from build123d import *

# Parameters (mm, degrees)
SKETCH1_R           = 1.905
BOSS_EXTRUDE1_DEPTH = 9.525
SKETCH2_R           = 45.72
CUT_EXTRUDE1_DEPTH  = 12.7
SKETCH4_R           = 1.905
CUT_EXTRUDE3_DEPTH  = 12.7
CIRPATTERN2_COUNT   = 4
SKETCH10_R          = 0.6985
CUT_EXTRUDE5_DEPTH  = 3.175
CIRPATTERN5_COUNT   = 4
CHAMFER1_SIZE       = 12.7
CHAMFER1_SIZE2      = 7.332348419


with BuildPart() as part:
    # Sketch1 → Boss-Extrude1 (new body)
    with BuildSketch(Plane(origin=(0, 0, 0), x_dir=(1, 0, 0), z_dir=(0, 1, 0))):
        with BuildLine():
            ThreePointArc((-66.860826677, 58.590441679), (-88.9, 0), (-66.860826677, -58.590441679))
            ThreePointArc((-66.860826677, -58.590441679), (-65.466067123, -65.466067123), (-58.590441679, -66.860826677))
            ThreePointArc((-58.590441679, -66.860826677), (0, -88.9), (58.590441679, -66.860826677))
            ThreePointArc((58.590441679, -66.860826677), (65.466067123, -65.466067123), (66.860826677, -58.590441679))
            ThreePointArc((66.860826677, -58.590441679), (88.9, 0), (66.860826677, 58.590441679))
            ThreePointArc((66.860826677, 58.590441679), (65.466067123, 65.466067123), (58.590441679, 66.860826677))
            ThreePointArc((58.590441679, 66.860826677), (0, 88.9), (-58.590441679, 66.860826677))
            ThreePointArc((-58.590441679, 66.860826677), (-65.466067123, 65.466067123), (-66.860826677, 58.590441679))
        make_face()
        with Locations(Location((-60.975939062, 60.975939062, 0), (0, 0, 90))):
            Circle(SKETCH1_R, mode=Mode.SUBTRACT)
        with Locations(Location((60.975939062, 60.975939062, 0), (0, 0, 90))):
            Circle(SKETCH1_R, mode=Mode.SUBTRACT)
        with Locations(Location((60.975939062, -60.975939062, 0), (0, 0, 90))):
            Circle(SKETCH1_R, mode=Mode.SUBTRACT)
        with Locations(Location((-60.975939062, -60.975939062, 0), (0, 0, 90))):
            Circle(SKETCH1_R, mode=Mode.SUBTRACT)
    extrude(amount=BOSS_EXTRUDE1_DEPTH)

    # Sketch2 → Cut-Extrude1 (cut)
    with BuildSketch(Plane(origin=(0, 9.525, 0), x_dir=(1, 0, 0), z_dir=(0, 1, 0))):
        with Locations(Location((0, 0, 0), (0, 0, 270))):
            Circle(SKETCH2_R)
    extrude(amount=-CUT_EXTRUDE1_DEPTH, mode=Mode.SUBTRACT)

    # Sketch4 → Cut-Extrude3 (cut)
    with BuildSketch(Plane(origin=(0, 9.525, 0), x_dir=(1, 0, 0), z_dir=(0, 1, 0))):
        with Locations(Location((0, 82.55, 0), (0, 0, 270))):
            Circle(SKETCH4_R)
    cut_extrude3 = extrude(amount=-CUT_EXTRUDE3_DEPTH, mode=Mode.SUBTRACT)

    # CirPattern2: Cut-Extrude3 ×4 about axis
    cirpattern2_axis = Axis((0, 0, 0), (0, 1, 0))
    for i in range(1, CIRPATTERN2_COUNT):
        add(cut_extrude3.rotate(cirpattern2_axis, i * 360 / CIRPATTERN2_COUNT), mode=Mode.SUBTRACT)

    # Sketch10 → Cut-Extrude5 (cut)
    with BuildSketch(Plane(origin=(-62.861792847, 0, -62.861792847), x_dir=(0, -1, 0), z_dir=(-0.7071067811865464, 0, -0.7071067811865488))):
        with Locations(Location((-4.826, 0, 0), (0, 0, 90))):
            Circle(SKETCH10_R)
    cut_extrude5 = extrude(amount=-CUT_EXTRUDE5_DEPTH, mode=Mode.SUBTRACT)

    # CirPattern5: Cut-Extrude5 ×4 about axis
    cirpattern5_axis = Axis((0, 0, 0), (0, 1, 0))
    for i in range(1, CIRPATTERN5_COUNT):
        add(cut_extrude5.rotate(cirpattern5_axis, i * 360 / CIRPATTERN5_COUNT), mode=Mode.SUBTRACT)

    # Chamfer1
    chamfer1_edges = [part.edges().sort_by_distance(p)[0] for p in [
        (0, 9.525, -45.72),
    ]]
    chamfer1_side = [part.faces().sort_by_distance(p)[0] for p in [
        (0, 9.525, -86.385528286),
    ]]
    chamfer(chamfer1_edges, length=CHAMFER1_SIZE, length2=CHAMFER1_SIZE2, reference=chamfer1_side[0])


solid = part.part
Read the model definition and answer for the solid it produces. Units are mm, in the model's axes. Coordinates: 2 decimals unless noted, no trailing zeros. Use a Markdown table: item, result.
Q1. Straight lines are drawn through the part: L1, parallel to X at y = 6, z = 61.5; L2, parallel to Z at x = -17.5, y = 4.25; L3, parallel to Z at x = 34.5, y = 1.25. For each, find the intervals that lie inside material, in ascending order. Write a range as [from, to].
Answer block:
| item | result |
|---|---|
| L1 | x = [-67.3, -62.81], [-59.14, 59.14], [62.81, 67.3] |
| L2 | z = [-87.16, -46.07], [46.07, 87.16] |
| L3 | z = [-81.93, -30], [30, 81.93] |
Q2. Determine the mould class of faces 1 (the face through (88.895, 4.696, 0.896)), 2 (the face through (13.92, 2.55, 44.2)), 3 (the face through (-88.895, 4.696, -0.896)), 4 (the face through (58, 9.525, 19)) for opening direction X: released by +X, released by -X, zero draft, split by the parting line, or undercut.
Answer block:
| item | result |
|---|---|
| face 1 | released by +X |
| face 2 | undercut |
| face 3 | released by -X |
| face 4 | zero draft |
Q3. Each of these flat-tipped pins is pushed along its axis until it touches: pin 1 Ø3.5 at (x, z) = (82.55, 0) entering from -Y; pin 2 Ø2 at (x, y) = (32, 8) entering from +Z; pin 3 Ø1 at (y, z) = (4.5, -44.5) entering from +X. Where does it stop, or does it pass through?
Answer block:
| item | result |
|---|---|
| pin 1 | passes through |
| pin 2 | stops at z = 83.32 |
| pin 3 | stops at x = 77.25 |
